Source: three-view drawing plus pictorial views. Frame: mm from the lowest corner of the part. Coordinates: 2 decimals unless noted, no trailing zeros. Loops run counter-clockwise (first coordinate to the right, second up) from the corner with the lowest first, then second, coordinate; pieces in that order, holes last. Notation, with made-up numbers: M 49.5,-35.5 L 77.5,-35.5 A25 ccw 77.5,-11.5 Z; hole C 24,-33.5 d4. An arc over 180 degrees is marked long. Write each question's results on one line, items separated by ' | '. Start each with the question number.
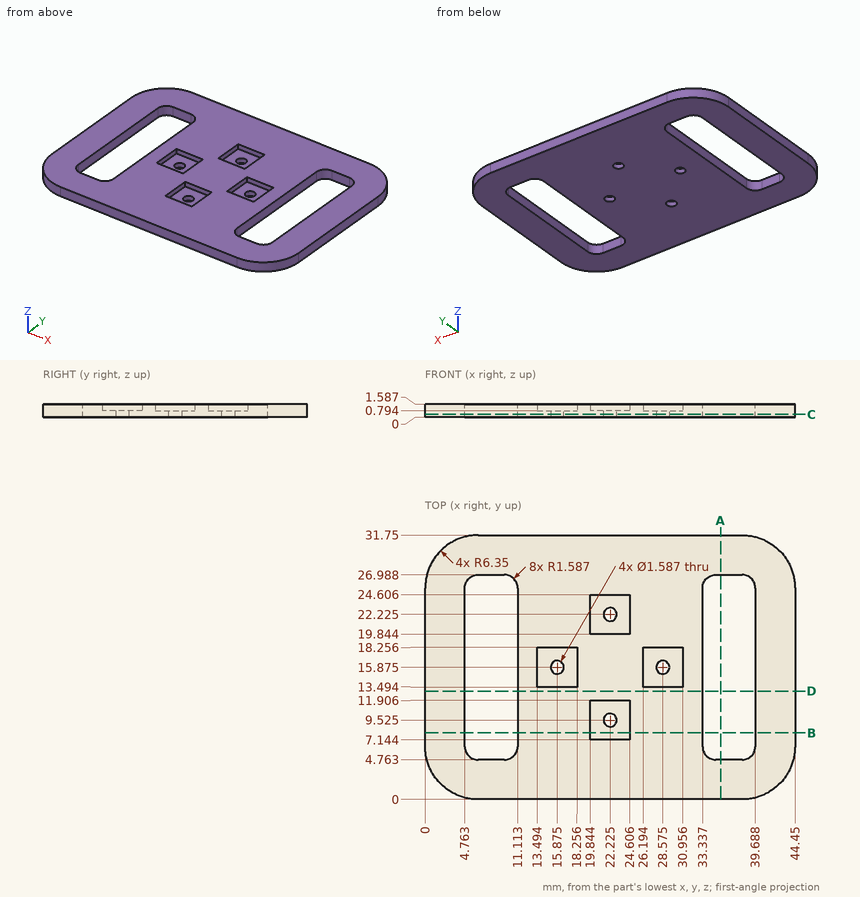
Item 1: Ray query, L1, parallel to X at y = 18, z = 0.7; L2, parallel to Y at x = 22, z = 0.9; L3, parallel to X at y = 10.5, z = 1. Return the intervals inside material, ascending. Write a range as [from, to].
Item 2: Section B-B, the plane y = 8. Return loops of the section in (x, z).
Item 3: Section D-D, the plane y = 13. Return loops of the section in (x, z).
Item 4: Contact query for a flat-ended pin moving along its axis: P1, Ø2.5, axis at x = 23, y = 10, coming from the +Z side. Output: stop coordinate, or through.
Item 5: Section A-A, the plane x = 35.5. Return loops of the section in (y, z), plus the area to 3 significant figures.
Item 6: Section C-C, the plane z = 0.35. Count the separate pieces of the cut face and the enclosed holes in it, plus the area to 3 significant figures.
Solutions:
1) L1: x = [0, 4.76], [11.11, 33.34], [39.69, 44.45] | L2: y = [0, 7.14], [11.91, 19.84], [24.61, 31.75] | L3: x = [0, 4.76], [11.11, 19.84], [24.61, 33.34], [39.69, 44.45]
2) outline: M 0,0 L 4.76,0 L 4.76,1.59 L 0,1.59 Z; M 11.11,0 L 33.34,0 L 33.34,1.59 L 24.61,1.59 L 24.61,0.79 L 19.84,0.79 L 19.84,1.59 L 11.11,1.59 Z; M 39.69,0 L 44.45,0 L 44.45,1.59 L 39.69,1.59 Z
3) outline: M 0,0 L 4.76,0 L 4.76,1.59 L 0,1.59 Z; M 11.11,0 L 33.34,0 L 33.34,1.59 L 11.11,1.59 Z; M 39.69,0 L 44.45,0 L 44.45,1.59 L 39.69,1.59 Z
4) P1: stops at z = 0.79
5) outline: M 0,0 L 4.76,0 L 4.76,1.59 L 0,1.59 Z; M 26.99,0 L 31.75,0 L 31.75,1.59 L 26.99,1.59 Z | area: 15.1 mm²
6) separate pieces: 1 | enclosed holes: 6 | area: 1,090 mm²
